Build history of the part. All positions in model axes, mm. A direction names the side the tool comes from. Round coordinates to 2 decimals unless told otherwise and drop trailing zeros. Write each loop counter-clockwise with the first axis right and the second up, starting at its lowest first coordinate (ties: lowest second). Pieces come first, ordered by that corner, then holes.
from build123d import *

# Parameters (mm, degrees)
F0_R         = 7
F1_DEPTH     = 70
F2_DEPTH     = 62
F3_R         = 5.5
F4_DEPTH     = 20
F6_DEPTH     = 8
F7_T4_ANGLE  = 59.9999999128
F7_T10_ANGLE = 59.9999996333
F7_T16_ANGLE = 60.0000004539
F7_T22_ANGLE = 59.9999999128
F7_T28_ANGLE = 60.0000002811
F7_T34_ANGLE = 59.9999998061


# Not quite as in the source:
# - a fillet or chamfer that OpenCascade refuses, or shapes differently, is made with other operations: its cross-section is extruded or revolved along the edge and cut away or added


with BuildPart() as f1:
    # F0 (on Front) → F1 (new body)
    with BuildSketch(Plane.XZ):
        Circle(F0_R)
        Polygon((2.7500007272, 4.7631393009), (5.5, 3.1754264805), (5.5, 0), (5.5, -3.1754264805), (2.7499994424, -4.7631400427), (0, -6.3508529611), (-2.7500008008, -4.7631392585), (-5.5, -3.1754264805), (-5.5, 0), (-5.5, 3.1754264805), (-2.7500002446, 4.7631395796), (0, 6.3508529611), align=None, mode=Mode.SUBTRACT)
    extrude(amount=F1_DEPTH)

    # F0 (on Front) → F2 (join)
    with BuildSketch(Plane.XZ):
        with BuildLine():
            Line((5.5, -3.1754264805), (5.5, 0))
            ThreePointArc((5.5, 0), (4.7631395599, -2.7500002788), (2.7499994424, -4.7631400427))
            Line((2.7499994424, -4.7631400427), (5.5, -3.1754264805))
        make_face()
        with BuildLine():
            Line((0, -6.3508529611), (2.7499994424, -4.7631400427))
            ThreePointArc((2.7499994424, -4.7631400427), (-7.842e-07, -5.5), (-2.7500008008, -4.7631392585))
            Line((-2.7500008008, -4.7631392585), (0, -6.3508529611))
        make_face()
        with BuildLine():
            Line((-5.5, -3.1754264805), (-2.7500008008, -4.7631392585))
            ThreePointArc((-2.7500008008, -4.7631392585), (-4.763139952, -2.7499995996), (-5.5, 0))
            Line((-5.5, 0), (-5.5, -3.1754264805))
        make_face()
        with BuildLine():
            ThreePointArc((-5.5, 0), (-4.7631397914, 2.7499998777), (-2.7500002446, 4.7631395796))
            Line((-2.7500002446, 4.7631395796), (-5.5, 3.1754264805))
            Line((-5.5, 3.1754264805), (-5.5, 0))
        make_face()
        with BuildLine():
            ThreePointArc((-2.7500002446, 4.7631395796), (2.787e-07, 5.5), (2.7500007272, 4.7631393009))
            Line((2.7500007272, 4.7631393009), (0, 6.3508529611))
            Line((0, 6.3508529611), (-2.7500002446, 4.7631395796))
        make_face()
        with BuildLine():
            Line((5.5, 0), (5.5, 3.1754264805))
            Line((5.5, 3.1754264805), (2.7500007272, 4.7631393009))
            ThreePointArc((2.7500007272, 4.7631393009), (4.7631399308, 2.7499996364), (5.5, 0))
        make_face()
    extrude(amount=F2_DEPTH)

    # F3 (on face) → F4 (join)
    with BuildSketch(Plane(origin=(0, 0, 0), x_dir=(-1, 0, 0), z_dir=(0, 1, 0))):
        with BuildLine():
            Line((-7, 0), (-7, -4.0414518843))
            Line((-7, -4.0414518843), (-3.5000000457, -6.0621778001))
            ThreePointArc((-3.5000000457, -6.0621778001), (-6.0621778397, -3.4999999772), (-7, 0))
        make_face()
        with BuildLine():
            Line((-7, 4.0414518843), (-7, 0))
            ThreePointArc((-7, 0), (-6.0621778147, 3.5000000204), (-3.4999999591, 6.0621778501))
            Line((-3.4999999591, 6.0621778501), (-7, 4.0414518843))
        make_face()
        with BuildLine():
            ThreePointArc((-3.4999999591, 6.0621778501), (-6.0621778147, 3.5000000204), (-7, 0))
            ThreePointArc((-7, 0), (-6.0621778397, -3.4999999772), (-3.5000000457, -6.0621778001))
            ThreePointArc((-3.5000000457, -6.0621778001), (-3.61e-08, -7), (3.4999999831, -6.0621778362))
            ThreePointArc((3.4999999831, -6.0621778362), (6.0621778216, -3.5000000084), (7, 0))
            ThreePointArc((7, 0), (6.06217782, 3.5000000113), (3.4999999774, 6.0621778395))
            ThreePointArc((3.4999999774, 6.0621778395), (1.05e-08, 7), (-3.4999999591, 6.0621778501))
        make_face()
        Circle(F3_R, mode=Mode.SUBTRACT)
        with BuildLine():
            ThreePointArc((3.4999999831, -6.0621778362), (-3.61e-08, -7), (-3.5000000457, -6.0621778001))
            Line((-3.5000000457, -6.0621778001), (0, -8.0829037687))
            Line((0, -8.0829037687), (3.4999999831, -6.0621778362))
        make_face()
        with BuildLine():
            Line((0, 8.0829037687), (-3.4999999591, 6.0621778501))
            ThreePointArc((-3.4999999591, 6.0621778501), (1.05e-08, 7), (3.4999999774, 6.0621778395))
            Line((3.4999999774, 6.0621778395), (0, 8.0829037687))
        make_face()
        with BuildLine():
            ThreePointArc((7, 0), (6.0621778216, -3.5000000084), (3.4999999831, -6.0621778362))
            Line((3.4999999831, -6.0621778362), (7, -4.0414518843))
            Line((7, -4.0414518843), (7, 0))
        make_face()
        with BuildLine():
            Line((7, 4.0414518843), (3.4999999774, 6.0621778395))
            ThreePointArc((3.4999999774, 6.0621778395), (6.06217782, 3.5000000113), (7, 0))
            Line((7, 0), (7, 4.0414518843))
        make_face()
    extrude(amount=F4_DEPTH)

    # F5 (on face) → F6 (cut, through all)
    with BuildSketch(Plane.XZ.offset(70)):
        with BuildLine():
            Line((5.5, 3.1754264805), (5.5, -3.1754264805))
            Line((5.5, -3.1754264805), (5.869161212, -3.814832456))
            ThreePointArc((5.869161212, -3.814832456), (6.7113384837, -1.9894561463), (7, 0))
            ThreePointArc((7, 0), (6.7113384837, 1.9894561463), (5.869161212, 3.814832456))
            Line((5.869161212, 3.814832456), (5.5, 3.1754264805))
        make_face()
        with BuildLine():
            Line((5.869161212, -3.814832456), (5.5, -3.1754264805))
            Line((5.5, -3.1754264805), (0, -6.3508529611))
            Line((0, -6.3508529611), (0.369161212, -6.9902589365))
            ThreePointArc((0.369161212, -6.9902589365), (3.5, -6.0621778265), (5.869161212, -3.814832456))
        make_face()
    extrude(amount=-F6_DEPTH, mode=Mode.SUBTRACT)

    # F7: chamfer of 1 on 6 edges, made by hand


with BuildPart() as f7_tool2:
    # F7_s3 → F7_t4 (revolve)
    with BuildSketch(Plane.XY):
        Polygon((-7, -1), (-8, 0), (-7, 0), align=None)
    revolve(axis=Axis((0, 0, 0), (0, -1, 0)), revolution_arc=F7_T4_ANGLE)

    split(bisect_by=Plane.YZ.offset(-7), keep=Keep.TOP)

    split(bisect_by=Plane(origin=(-3.5, 0, -6.0621778265), x_dir=(0, 1, 0), z_dir=(0.5, 0, 0.8660254038)), keep=Keep.TOP)


with BuildPart() as f1_1:
    add(f1.part)

    # F7_t1: union F7_tool2
    add(f7_tool2.part)


with BuildPart() as f7_tool8:
    # F7_s9 → F7_t10 (revolve)
    with BuildSketch(Plane.XY):
        Polygon((7, -1), (8, 0), (7, 0), align=None)
    revolve(axis=Axis((0, 0, 0), (0, -1, 0)), revolution_arc=F7_T10_ANGLE)

    split(bisect_by=Plane(origin=(3.5, 0, 6.0621778265), x_dir=(0, 1, 0), z_dir=(-0.5, 0, -0.8660254038)), keep=Keep.TOP)

    split(bisect_by=Plane.YZ.offset(7), keep=Keep.BOTTOM)


with BuildPart() as f1_2:
    add(f1_1.part)

    # F7_t7: union F7_tool8
    add(f7_tool8.part)


with BuildPart() as f7_tool14:
    # F7_s15 → F7_t16 (revolve)
    with BuildSketch(Plane(origin=(0, 0, 0), x_dir=(0, 1, 0), z_dir=(0.8660254006, 0, -0.5000000055))):
        Polygon((-1, 7), (0, 8), (0, 7), align=None)
    revolve(axis=Axis((0, 0, 0), (0, -1, 0)), revolution_arc=F7_T16_ANGLE)

    split(bisect_by=Plane(origin=(3.5, 0, 6.0621778265), x_dir=(0, 1, 0), z_dir=(-0.5, 0, -0.8660254038)), keep=Keep.TOP)

    split(bisect_by=Plane(origin=(-3.5, 0, 6.0621778265), x_dir=(0, 1, 0), z_dir=(0.5, 0, -0.8660254038)), keep=Keep.TOP)


with BuildPart() as f1_3:
    add(f1_2.part)

    # F7_t13: union F7_tool14
    add(f7_tool14.part)


with BuildPart() as f7_tool20:
    # F7_s21 → F7_t22 (revolve)
    with BuildSketch(Plane(origin=(0, 0, 0), x_dir=(0, 1, 0), z_dir=(0.866025403, 0, 0.5000000013))):
        Polygon((-1, 7), (0, 8), (0, 7), align=None)
    revolve(axis=Axis((0, 0, 0), (0, -1, 0)), revolution_arc=F7_T22_ANGLE)

    split(bisect_by=Plane(origin=(-3.5, 0, 6.0621778265), x_dir=(0, 1, 0), z_dir=(0.5, 0, -0.8660254038)), keep=Keep.TOP)

    split(bisect_by=Plane.YZ.offset(-7), keep=Keep.TOP)


with BuildPart() as f1_4:
    add(f1_3.part)

    # F7_t19: union F7_tool20
    add(f7_tool20.part)


with BuildPart() as f7_tool26:
    # F7_s27 → F7_t28 (revolve)
    with BuildSketch(Plane(origin=(0, 0, 0), x_dir=(0, 1, 0), z_dir=(-0.866025403, 0, 0.5000000013))):
        Polygon((-1, 7), (0, 8), (0, 7), align=None)
    revolve(axis=Axis((0, 0, 0), (0, -1, 0)), revolution_arc=F7_T28_ANGLE)

    split(bisect_by=Plane(origin=(3.5, 0, -6.0621778265), x_dir=(0, 1, 0), z_dir=(-0.5, 0, 0.8660254038)), keep=Keep.TOP)

    split(bisect_by=Plane(origin=(-3.5, 0, -6.0621778265), x_dir=(0, 1, 0), z_dir=(0.5, 0, 0.8660254038)), keep=Keep.TOP)


with BuildPart() as f1_5:
    add(f1_4.part)

    # F7_t25: union F7_tool26
    add(f7_tool26.part)


with BuildPart() as f7_tool32:
    # F7_s33 → F7_t34 (revolve)
    with BuildSketch(Plane(origin=(0, 0, 0), x_dir=(0, 1, 0), z_dir=(-0.8660254021, 0, -0.5000000029))):
        Polygon((-1, 7), (0, 8), (0, 7), align=None)
    revolve(axis=Axis((0, 0, 0), (0, -1, 0)), revolution_arc=F7_T34_ANGLE)

    split(bisect_by=Plane(origin=(3.5, 0, -6.0621778265), x_dir=(0, 1, 0), z_dir=(-0.5, 0, 0.8660254038)), keep=Keep.TOP)

    split(bisect_by=Plane.YZ.offset(7), keep=Keep.BOTTOM)


with BuildPart() as f1_6:
    add(f1_5.part)

    # F7_t31: union F7_tool32
    add(f7_tool32.part)


solid = f1_6.part
1) Mould opens along X. For faces 1 (the flat face through (-5.5, -66, 0)), 2 (the conical face through (0, -0.7, -7.3)), 3 (the flat face through (0, -62, 6)) say: released by +X, released by -X, zero draft, split by the parting line, or undercut.
Results:
face 1: released by +X
face 2: split by the parting line
face 3: undercut
2) Wall check: L1, parallel to Z at x = 0, y = 6; L2, parallel to X at y = 6, z = 0. Give the ranges that are in metal, low to high.
Results:
L1: z = -8.08 to -5.5, 5.5 to 8.08
L2: x = -7 to -5.5, 5.5 to 7
3) Slice it at B-B (y = -30). Write the cut outline in (x, z).
Results:
outline: circle Ø14 at (0, 0); hole circle Ø11 at (0, 0)
4) Pin check, flat tips, straight feed: pin 1 Ø3 at (x, z) = (0.5, -4) entering from -Y; pin 2 Ø5 at (x, y) = (0.5, -7.5) entering from +Z; pin 3 Ø2 at (x, y) = (4, 9.5) entering from -Z. Stop position of each tip, or through.
Results:
pin 1: stops at y = -62
pin 2: stops at z = 7
pin 3: stops at z = -6.35
5) Which spindle directions (+Z, -Z, +X, -X, +Y, -Y) get a long thin tool onto all of the face, cutting with end or side? Do faces 4 (the flat face through (-5, -62, -3)), 5 (the cylindrical face through (-5.16, -35.02, 4.73)), 6 (the flat face through (5, 20, -3)). Say none if no direction does.
Results:
face 4: +X, -Y
face 5: -Y
face 6: +Z, -Z, +X, -X, +Y
6) Slice it at A-A (y = 10). Write the cut outline in (x, z), plus the area to 3 significant figures.
Results:
outline: (-7, -4.04) - (0, -8.08) - (7, -4.04) - (7, 4.04) - (0, 8.08) - (-7, 4.04) - close; hole circle Ø11 at (0, 0)
area: 74.7 mm2
